Solid Edge part; units mm, degrees
sketch "Sketch1" plane through (0, 0, 0) normal (0, -1, 0) x (1, 0, 0)
  line L0 (20, 20) -> (-20, 20)
  line L1 (-20, 20) -> (-18.949, 10)
  line L2 (-18.949, 10) -> (-11.1803, 10)
  line L3 (15, 0) -> (20, 0)
  line L4 (20, 0) -> (20, 20)
  arc A0 (-11.1803, 10) -> (15, 0) centre (0, 0) cw
extrude "Protrusion1" add sketch "Sketch1" against normal blind 63
sketch "Sketch2" plane through (20, 31.5, 10) normal (1, 0, 0) x (0, 1, 0)
  line L0 (31.5, -10) -> (25.5, -10)
  line L1 (25.5, -10) -> (24.2388, -1.0258)
  arc A0 (17.3069, 5) -> (24.2388, -1.0258) centre (17.3069, -2) cw
  line L2 (0, 5) -> (17.3069, 5)
  line L3 (0, 5) -> (-17.6206, 5)
  arc A1 (-17.6206, 5) -> (-24.5823, -1.2683) centre (-17.6206, -2) ccw
  line L4 (-25.5, -10) -> (-24.5823, -1.2683)
  line L5 (-31.5, -10) -> (-25.5, -10)
extrude "Recorte_Extrudado_1" cut sketch "Sketch2" against normal blind 40 material side at (20, 60, -0.05)
hole "Furo_1" at (14, 21.5, 20) direction (0, 0, -1) diameter 4 depth 10
hole "Hole1" at (14, 41.5, 20) direction (0, 0, -1) diameter 4 depth 10
hole "Hole2" at (-15.5, 4, 20) direction (0, 0, -1) diameter 4 depth 10
hole "Hole3" at (-15.5, 59, 20) direction (0, 0, -1) diameter 4 depth 10
hole "Furo_8" at (0, 31.5, 20) direction (0, 0, -1) diameter 7 depth 10
hole "Furo_9" at (0, 9.5, 20) direction (0, 0, -1) diameter 4 end up to next
hole "Hole4" at (0, 53.5, 20) direction (0, 0, -1) diameter 4 end up to next
properties material "PVC"
Can you work these out from the model? Positions are in its coordinate system, mm. A direction names the side the tool comes from. Coordinates: 2 decimals unless noted, no trailing zeros. Loops run counter-clockwise (first coordinate to the right, second up) from the corner with the lowest first, then second, coordinate; pieces in that order, holes last. Notation, with made-up numbers: M 63,51.25 L 98,51.25 A12 ccw 98,68.25 Z; hole C 42,-33 d8. An arc over 180 degrees is marked long. Answer as CSV lines item,"result". Start each with the question number.
1. Suppose I cut it at B-B, the plane x = -15.5. List the corners of the cut face in (y, z) for me, plus the area to 3 significant figures.
2. Thinking about a two-plate mould opening in X: for faces 1 (the face through (-1.2, 11.1, 17.5)), 2 (the face through (-19.6, 31.1, 16.2)), 3 (the face through (12.648, 22.974, 17.465)), 4 (the face through (1, 27, 15)), which applies, +X half, -X half, draft (parallel to the pull), parting line (faces both ways), or undercut?
3. Suppose I cut it at A-A, the plane y = 41.5. List the corners of the cut face in (x, z) for me.
4. Suppose I cut it at D-D, the plane y = 31.5. List the corners of the cut face in (x, z) for me.
5. For faces 5 (the face through (12.36, 10.16, 13.93)), 6 (the face through (5, 31, 20)), which set-ups out of +Z, -Z, +X, -X, +Y, -Y let a thin tool reach every point of the face, with its end or its side?
6. Suppose I cut it at C-C, the plane z = 13.25. List the corners of the cut face in (x, y) for me.
7. If I drill on probe 1 along Y at (x, z) = (0, 17); probe 2 along Y at (x, z) = (-15.5, 15.75); probe 3 along X at (y, z) = (57.5, 10.5), over which ranges is the centre line in solid material (lowest first)? Write a range as [from, to].
8. For pin 1 Ø3.5 at (x, y) = (-14, 60) entering from -Z; pin 2 Ø10 at (y, z) = (22.5, 17.5) entering from -X; pin 3 Ø6.5 at (x, y) = (14, 41.5) entering from -Z, each with a flat end and sliding along its axis, tell me the tip position at first contact or that it passes through.
Output:
1,outline,"M 0,10 L 2,10 L 2,20 L 0,20 Z; M 6,10 L 7.17,10 A7 cw 13.88,15 L 48.81,15 A7 cw 55.52,10 L 57,10 L 57,20 L 6,20 Z; M 61,10 L 63,10 L 63,20 L 61,20 Z"
1,area,"326 mm^2"
2,face 1,"undercut"
2,face 2,"-X half"
2,face 3,"undercut"
2,face 4,"draft"
3,outline,"M -20,20 L -19.47,15 L 12,15 L 12,20 Z; M 16,15 L 20,15 L 20,20 L 16,20 Z"
4,outline,"M -20,20 L -19.47,15 L -3.5,15 L -3.5,20 Z; M 3.5,15 L 20,15 L 20,20 L 3.5,20 Z"
5,face 5,"-Z, +X, -X"
5,face 6,"+Z, +X, -X, +Y, -Y"
6,outline,"M -19.29,0 L -7.03,0 L -7.03,9.25 L -19.29,9.25 Z; M -19.29,53.44 L -7.03,53.44 L -7.03,63 L -19.29,63 Z; M 7.03,0 L 20,0 L 20,9.25 L 7.03,9.25 Z; M 7.03,53.44 L 20,53.44 L 20,63 L 7.03,63 Z; hole C -15.5,4 d4; hole C -15.5,59 d4"
7,probe 1,"y = [0, 7.5], [11.5, 28], [35, 51.5], [55.5, 63]"
7,probe 2,"y = [0, 2], [6, 57], [61, 63]"
7,probe 3,"x = [-19, -16.82], [-14.18, -10.71], [10.71, 20]"
8,pin 1,"stops at z = 10"
8,pin 2,"stops at x = -20"
8,pin 3,"stops at z = 15"
